Autodesk Inventor part; units mm, degrees
ref_plane "YZ Plane" through (0, 0, 0) normal (1, 0, 0) x (0, 1, 0)
ref_plane "XZ Plane" through (0, 0, 0) normal (0, 1, 0) x (-1, 0, 0)
ref_plane "XY Plane" through (0, 0, 0) normal (0, 0, 1) x (1, 0, 0)
sketch "Sketch1" plane through (0, 0, 0) normal (0, 1, 0) x (-1, 0, 0)
  line L0 (0, 0) -> (22, 0)
  line L1 (22, 0) -> (22, -22)
  line L2 (22, -22) -> (0, -22)
  line L3 (0, -22) -> (0, 0)
  dimension "d0" = 22
  dimension "d1" = 22
extrude "Extrusion1" add sketch "Sketch1" along normal blind 55
ref_plane "Work Plane1" through (-11, 0, 0) normal (1, 0, 0) x (0, 0, -1)
sketch "Sketch2" plane through (-11, 0, 0) normal (1, 0, 0) x (0, 0, -1)
  line L0 (0, 55) -> (22, 55)
  line L1 (11, 55) -> (9, 55)
  line L2 (22, 55) -> (0, 55)
  line L3 (9, 55) -> (9, 64)
  line L4 (9, 64) -> (3, 64)
  line L5 (3, 64) -> (3, 68)
  line L6 (3, 68) -> (9, 68)
  line L7 (9, 68) -> (9, 74)
  line L8 (9, 74) -> (13, 74)
  line L9 (13, 74) -> (13, 68)
  line L10 (13, 68) -> (19, 68)
  line L11 (19, 68) -> (19, 64)
  line L12 (19, 64) -> (13, 64)
  line L13 (13, 64) -> (13, 55)
  point P0 (0, 0)
  dimension "d4" = 2
  dimension "d5" = 9
  dimension "d6" = 6
  dimension "d7" = 4
  dimension "d8" = 6
  dimension "d9" = 4
  dimension "d10" = 6
extrude "Extrusion2" add sketch "Sketch2" along normal mid plane 4
properties part number "king"
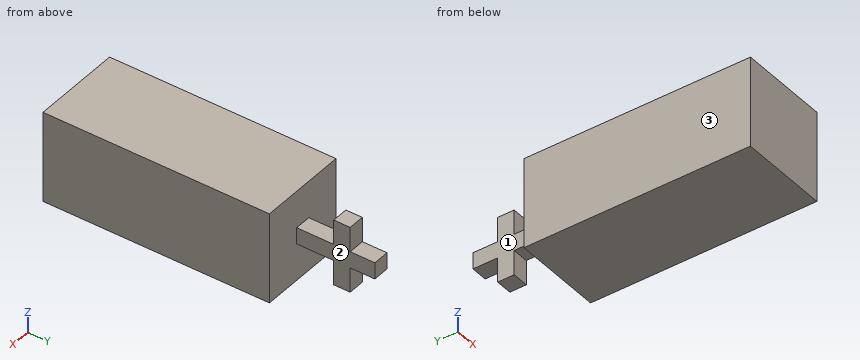
The listing builds one solid part. Answer for the finished solid, in the listing's coordinates (mm). Face numbers are marked on the shaded views. A direction names the side the tool comes from. Coordinates: 2 decimals unless noted, no trailing zeros. Write each loop counter-clockwise with the first axis right and the second up, starting at its lowest first coordinate (ties: lowest second). Pieces come first, ordered by that corner, then holes. Notation, with made-up numbers: (45.5, -13.75) - (91.5, -13.75) arc R17 cw to (91.5, 18.25) - close; hole circle Ø2 at (-39.5, 31). An arc over 180 degrees is marked (long way). Return JSON: item names as keys, results as strings.
1. The part is cut by section C-C on z = -11.75. Determine the outline of the cut face in (x, y), then the cut area to 3 significant figures.
Final values:
{"outline": "(-22, 0) - (0, 0) - (0, 55) - (-9, 55) - (-9, 74) - (-13, 74) - (-13, 55) - (-22, 55) - close", "area": "1,290 mm^2"}
2. Each of these flat-tipped pins is pushed along its axis until it touches: pin 1 Ø2 at (x, z) = (-11.5, -15) entering from +Y; pin 2 Ø4.5 at (x, y) = (-12, 58.5) entering from +Z; pin 3 Ø4.5 at (x, y) = (-12, 67) entering from +Z. Where does it stop, or does it pass through?
Final values:
{"pin 1": "y = 68", "pin 2": "z = -9", "pin 3": "z = -3"}
3. The part is cut by section D-D on x = -4. Determine the outline of the cut face in (y, z), then the cut area to 3 significant figures.
Final values:
{"outline": "(0, -22) - (55, -22) - (55, 0) - (0, 0) - close", "area": "1,210 mm^2"}
4. The part is cut by section A-A on z = -7.25. Determine the outline of the cut face in (x, y), then the cut area to 3 significant figures.
Final values:
{"outline": "(-22, 0) - (0, 0) - (0, 55) - (-22, 55) - close; (-13, 64) - (-9, 64) - (-9, 68) - (-13, 68) - close", "area": "1,230 mm^2"}
5. The part is cut by section B-B on y = 66.5. Determine the outline of the cut face in (x, z).
Final values:
{"outline": "(-13, -19) - (-9, -19) - (-9, -3) - (-13, -3) - close"}
6. Consider line 1 along Y through (x, z) = (-1, -17.5); line 2 along X through (y, z) = (68.5, -10.25). Determine where each line is inside the solid, lowest interval first.
Final values:
{"line 1": "0 to 55", "line 2": "-13 to -9"}
7. Which of the six approach directions +Z, -Z, +X, -X, +Y, -Y give full straight-line access (tool end or side, diameter ignored) to the marked faces 1, 2 and 3?
Final values:
{"face 1": "+Z, -Z, -X, +Y", "face 2": "+Z, -Z, +X, +Y", "face 3": "+Z, -Z, -X, +Y, -Y"}
